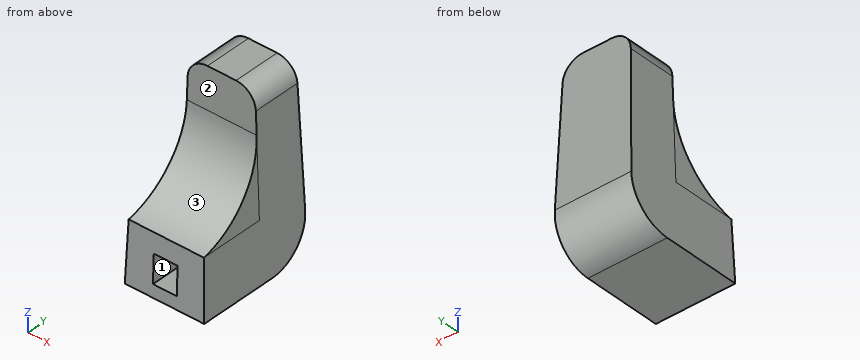
```python
from build123d import *

# Parameters (mm, degrees)
F0_W        = 20
F0_H        = 30
F1_DEPTH    = 45
F1_TAPER    = 2
F4_DEPTH    = 20.001
F5_T4_DEPTH = 116.9802704864
F7_W        = 6
F7_H        = 7
F8_DEPTH    = 10
F9_R        = 5
F10_R       = 10


# Not quite as in the source:
# - a fillet or chamfer that OpenCascade refuses, or shapes differently, is made with other operations: its cross-section is extruded or revolved along the edge and cut away or added


with BuildPart() as f1:
    # F0 (on Top) → F1 (new body)
    with BuildSketch(Plane.XY):
        Rectangle(F0_W, F0_H)
    extrude(amount=F1_DEPTH, taper=F1_TAPER)

    # F3 (on face) → F4 (cut, through all)
    with BuildSketch(Plane(origin=(-10, 0, 0), x_dir=(0, -1, 0), z_dir=(-1, 0, 0))):
        Polygon((14.4761884576, 15), (13.4285653729, 45), (-1.5714346271, 45), (-1.5714346271, 15), (13.4285653729, 15), align=None)
    extrude(amount=-F4_DEPTH, mode=Mode.SUBTRACT)

    # F5: fillet of radius 20 on 1 edges, made by hand


with BuildPart() as f5_tool2:
    # F5_s3 → F5_t4 (new body)
    with BuildSketch(Plane.YZ.offset(-58.4901352432)):
        with BuildLine():
            ThreePointArc((-14.4761884576, 15), (-2.9520099049, 21.9376573833), (1.5714346271, 34.6055787142))
            Line((1.5714346271, 34.6055787142), (1.5714346271, 15))
            Line((1.5714346271, 15), (-14.4761884576, 15))
        make_face()
    extrude(amount=F5_T4_DEPTH)

    split(bisect_by=Plane(origin=(-9.9878202513, 0, 0.3487823687), x_dir=(0, 1, 0), z_dir=(0.999390827, 0, -0.0348994967)), keep=Keep.TOP)

    split(bisect_by=Plane(origin=(9.9878202513, 0, 0.3487823687), x_dir=(0, 1, 0), z_dir=(-0.999390827, 0, -0.0348994967)), keep=Keep.TOP)


with BuildPart() as f1_1:
    add(f1.part)

    # F5_t1: union F5_tool2
    add(f5_tool2.part)

    # F7 (on face) → F8 (cut)
    with BuildSketch(Plane(origin=(0, -15, 0), x_dir=(-1, 0, 0), z_dir=(0, 1, 0))):
        with Locations((0, 6.6315173171)):
            Rectangle(F7_W, F7_H)
    extrude(amount=F8_DEPTH, mode=Mode.SUBTRACT)

    # F9
    f9_edges = [f1_1.edges().sort_by_distance(p)[0] for p in [
        (-8.428565, 7.5, 45),
        (8.428565, 7.5, 45),
    ]]
    fillet(f9_edges, radius=F9_R)

    # F10
    f10_edges = [f1_1.edges().sort_by_distance(p)[0] for p in [
        (0, 15, 0),
    ]]
    fillet(f10_edges, radius=F10_R)


solid = f1_1.part
```
Build history of the part. All positions in model axes, mm. Face numbers are marked on the shaded views. Round coordinates to 2 decimals unless told otherwise and drop trailing zeros. Loops run counter-clockwise (first coordinate to the right, second up) from the corner with the lowest first, then second, coordinate; pieces in that order, holes last. Notation, with made-up numbers: M 0,38.25 L 50,38.25 A24 ccw 50,54.25 Z; hole C 37.5,71.25 d3. An arc over 180 degrees is marked long. Answer as CSV lines item,"result".
1. Two-plate mould, pull along Z, no slides. Class the marked faces 1, 2 and 3: released by +Z, released by -Z, zero draft, split by the parting line, or undercut.
Resolved:
face 1,"undercut"
face 2,"zero draft"
face 3,"released by +Z"
2. Cut at D-D on y = 3.25. Write the cut outline in (x, z).
Resolved:
outline,"M -10,0 L 10,0 L 8.6,40.17 A5 ccw 3.6,45 L -3.6,45 A5 ccw -8.6,40.17 Z"
3. Cut at A-A on x = -1.5. Write the cut outline in (y, z), then the cut area to 3 significant figures.
Resolved:
outline,"M -15,0 L 4.64,0 A10 ccw 14.64,10.35 L 13.43,45 L 1.57,45 L 1.57,34.61 A20 cw -14.48,15 L -14.65,10.13 L -5,10.13 L -5,3.13 L -14.89,3.13 Z"
area,"801 mm²"
4. Cut at B-B on y = -9.5. Write the cut outline in (x, z), then the cut area to 3 significant figures.
Resolved:
outline,"M -10,0 L 10,0 L 9.42,16.71 L -9.42,16.71 Z; hole M -3,3.13 L 3,3.13 L 3,10.13 L -3,10.13 Z"
area,"282 mm²"
5. Cut at C-C on z = 8. Write the cut outline in (x, y).
Resolved:
outline,"M -9.72,-14.72 L -3,-14.72 L -3,-5 L 3,-5 L 3,-14.72 L 9.72,-14.72 L 9.72,14.44 L -9.72,14.44 Z"
6. Flat gauge pins, fed straight in: P1, Ø1.5, axis at x = -3, z = 28, coming from the +Y side; P2, Ø4, axis at y = 2, z = 16, coming from the +X side; P3, Ø8.5, axis at x = -2.5, z = 37.5, coming from the -Y side; P4, Ø12, axis at x = 5.5, z = 7.5, coming from the +Y side. Where does each tip first touch, or does it go through?
Resolved:
P1,"stops at y = 14.05"
P2,"stops at x = 9.51"
P3,"stops at y = 1.53"
P4,"stops at y = 14.64"
7. Wall check: probe 1 along Y at (x, z) = (-3.25, 10); probe 2 along X at (y, z) = (-11.5, 9); probe 3 along Z at (x, y) = (-4.5, 7). Give the ranges that are in metal, low to high. Write a range as [from, to].
Resolved:
probe 1,"y = [-14.65, 14.64]"
probe 2,"x = [-9.69, -3], [3, 9.69]"
probe 3,"z = [0.28, 44.92]"
